CAD build for the part. Positions are in the model's coordinates, mm. A direction names the side the tool comes from. Coordinates: 2 decimals unless noted, no trailing zeros. Order: outer loops, then holes, each group sorted by start corner. A loop starts at its lowest first (then second) coordinate and runs counter-clockwise, first axis right, second up. Notation, with made-up numbers: M 79.25,51 L 124.25,51 A26 cw 124.25,82 Z; hole C 43,87 d2. An arc over 180 degrees is marked long. Write item = value, one per line. Start each with the question number.
Autodesk Inventor part; units mm, degrees
ref_plane "YZ Plane" through (0, 0, 0) normal (1, 0, 0) x (0, 1, 0)
ref_plane "XZ Plane" through (0, 0, 0) normal (0, 1, 0) x (-1, 0, 0)
ref_plane "XY Plane" through (0, 0, 0) normal (0, 0, 1) x (1, 0, 0)
sketch "Sketch1" plane through (0, 0, 0) normal (0, 1, 0) x (-1, 0, 0)
  line L0 (0, 0) -> (25.4, 0)
  line L1 (25.4, 0) -> (25.4, -3.175)
  line L2 (25.4, -3.175) -> (3.175, -3.175)
  line L3 (3.175, -3.175) -> (3.175, -50.8)
  line L4 (3.175, -50.8) -> (0, -50.8)
  line L5 (0, -50.8) -> (0, 0)
  dimension "d0" = 25.4
  dimension "d1" = 50.8
  dimension "d2" = 3.175
  dimension "d3" = 3.175
extrude "Extrusion1" add sketch "Sketch1" along normal mid plane 18.9992
sketch "Sketch2" plane through (-25.4, 9.4996, 0) normal (0, 0, 1) x (1, 0, 0)
  line L0 (0, 0) -> (25.4, 0) construction
  line L1 (25.4, -18.9992) -> (25.4, 0) construction
  line L2 (0, 0) -> (25.4, -18.9992) construction
  line L3 (0, 0) -> (0, -18.9992) construction
  line L4 (0, -18.9992) -> (25.4, 0) construction
  point P0 (25.4, -9.4996)
  point P1 (12.7, -9.4996)
hole "Hole1" at (-12.7, 0, 0) direction (0, 0, -1) diameter 8.4328 end through all
sketch "Sketch3" plane through (0, -9.4996, -50.8) normal (1, 0, 0) x (0, 0, -1)
  line L0 (0, 18.9992) -> (0, 0) construction
  line L1 (-50.8, 18.9992) -> (-50.8, 0) construction
  line L2 (0, 0) -> (-50.8, 0) construction
  line L3 (-50.8, 9.4996) -> (0, 9.4996) construction
  point P0 (-38.1, 9.4996)
  point P1 (-25.4, 9.4996)
  point P2 (-12.7, 9.4996)
  dimension "d20" = 12.7
  dimension "d23" = 12.7
hole "Hole3" at (0, 0, -12.7) at (0, 0, -25.4) at (0, 0, -38.1) direction (-1, 0, 0) diameter 6.7564 end through all
properties part number "simpleBracketForTopOfDart"
1. Slice it at C-C (x = -12.7). Write the cut outline in (y, z) (3 decimals).
2. Flat gauge pins, fed straight in: pin 1 (9.5 mm diameter, centred on x = -12.7, y = 0, fed in from +Z); pin 2 (8 mm diameter, centred on y = 0, z = -12.7, fed in from -X) (3 decimals); pin 3 (4 mm diameter, centred on y = 0, z = -25.4, fed in from +X); pin 4 (6 mm diameter, centred on x = -11.5, y = -7, fed in from -Z) (3 decimals). Where does each tip first touch, or does it go through?
3. 3-axis set-ups, long thin cutter, end or side, ignore diameter. For faces 5 (the flat face through (-17, -2, -3.175)), 6 (the flat face through (-2, 9.5, -18)): which of +Z, -Z, +X, -X, +Y, -Y reach the whole face in a straight line?
4. Mould opens along Y. For faces 1 (the flat face through (-25.4, 0, -2)), 2 (the flat face through (-2, -9.5, -18)), 3 (the cylindrical face through (-1.61, -0.149, -22.025)), 4 (the cylindrical face through (-1.61, -1.015, -41.322)) say: released by +Y, released by -Y, zero draft, split by the parting line, or undercut.
5. Probe L1, parallel to Z at x = -0.85, y = 0; L2, parallel to Y at x = -12.7, z = -2.05; L3, parallel to Y at x = -2.3, z = -38.1. List the from-to ranges inside material, lowest first.
6. Slice it at A-A (z = -38.1). Write the cut outline in (x, y) (3 decimals).
7. Slice it at D-D (y = -5). Write the cut outline in (x, z) (3 decimals).
8. Slice it at B-B (y = 0). Write the cut outline in (x, z) (3 decimals).
Calculated:
q1.outline = M -9.5,-3.175 L -4.216,-3.175 L -4.216,0 L -9.5,0 Z; M 4.216,-3.175 L 9.5,-3.175 L 9.5,0 L 4.216,0 Z
q2.pin_1 = 0
q2.pin_2 = -3.175
q2.pin_3 = through
q2.pin_4 = -3.175
q3.face_5 = -Z, -X, +Y, -Y
q3.face_6 = +Z, -Z, +X, -X, +Y
q4.face_1 = zero draft
q4.face_2 = released by -Y
q4.face_3 = undercut
q4.face_4 = undercut
q5.L1 = -50.8 to -41.48, -34.72 to -28.78, -22.02 to -16.08, -9.32 to 0
q5.L2 = -9.5 to -4.22, 4.22 to 9.5
q5.L3 = -9.5 to -3.38, 3.38 to 9.5
q6.outline = M -3.175,-9.5 L 0,-9.5 L 0,-3.378 L -3.175,-3.378 Z; M -3.175,3.378 L 0,3.378 L 0,9.5 L -3.175,9.5 Z
q7.outline = M -25.4,-3.175 L -3.175,-3.175 L -3.175,-50.8 L 0,-50.8 L 0,0 L -25.4,0 Z
q8.outline = M -25.4,-3.175 L -16.916,-3.175 L -16.916,0 L -25.4,0 Z; M -8.484,-3.175 L -3.175,-3.175 L -3.175,-9.322 L 0,-9.322 L 0,0 L -8.484,0 Z; M -3.175,-50.8 L 0,-50.8 L 0,-41.478 L -3.175,-41.478 Z; M -3.175,-34.722 L 0,-34.722 L 0,-28.778 L -3.175,-28.778 Z; M -3.175,-22.022 L 0,-22.022 L 0,-16.078 L -3.175,-16.078 Z
